Input: dimensioned drawing with shaded views. Units: mm. Origin: part minimum x, y, z. A direction names the side the tool comes from. Round coordinates to 2 decimals unless told otherwise and drop trailing zeros. Loops run counter-clockwise (first coordinate to the right, second up) from the corner with the lowest first, then second, coordinate; pieces in that order, holes last. Notation, with made-up numbers: M -13,64 L 3,64 A15 ccw 3,84 Z; hole C -12,27 d10. An arc over 180 degrees is marked long. Write each question's results on one line, items separated by ' | '. Start each with the question number.
1. Set-up query: the marked faces 1, 2 and 3. Return all of +Z, -Z, +X, -X, +Y, -Y with unobstructed straight access to the full face (end or side cutting, diameter ignored); none if empty.
2. Section C-C on z = 12. Output: boundary loops of the cut face in (x, y).
3. Draft query along Y for the marked faces 4, 5 and 6. Return one class per face: released by +Y, released by -Y, zero draft, split by the parting line, or undercut.
4. Ray query, line 1 (X direction, y = 38, z = 14.5); line 2 (Y direction, x = 10.5, z = 7); line 3 (Y direction, x = 40, z = 13.5) (1 decimal). Return the intervals inside material, ascending.
5. Section A-A on y = 40. Output: boundary loops of the cut face in (x, z).
6. Section D-D on y = 11. Output: boundary loops of the cut face in (x, z), and give its area (3 significant figures).
7. Contact query for flat-ended pins moving along their axis: pin 1 Ø10 at (x, y) = (37.13, 40) entering from -Z; pin 2 Ø3 at (x, z) = (19, 6.5) entering from -Y. Output: stop coordinate, or through.
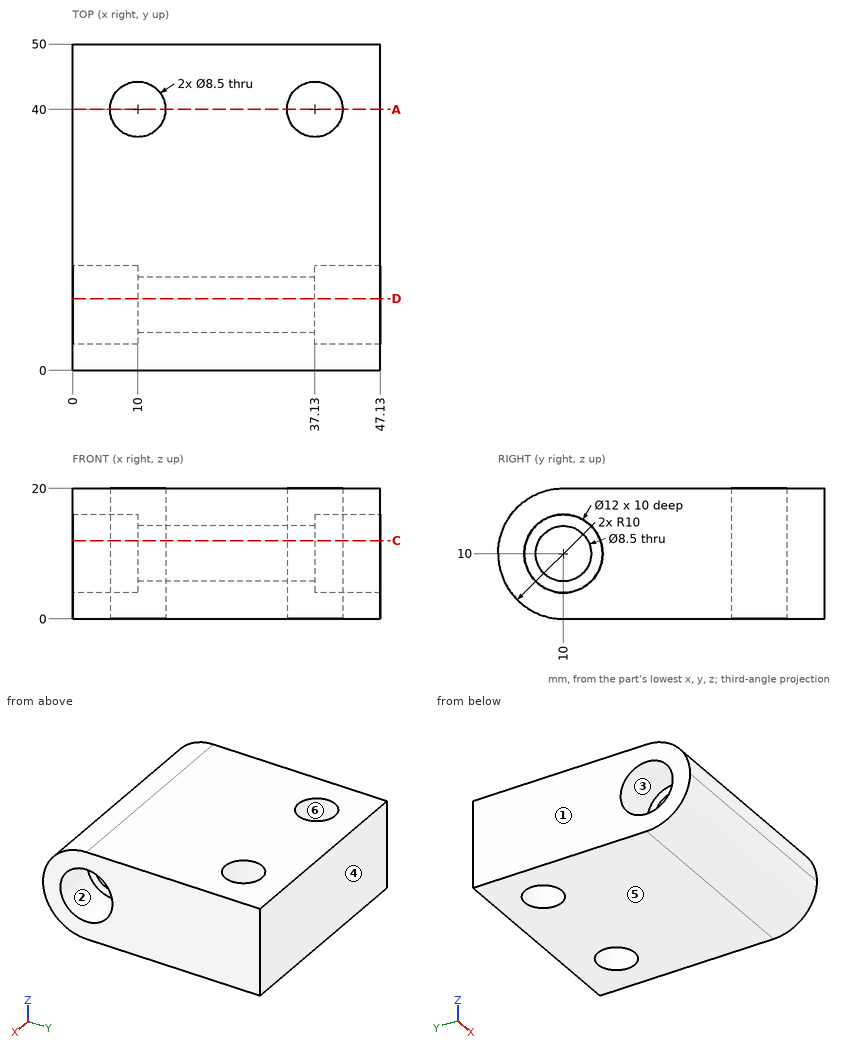
Taken from the geometry:
1) face 1: +Z, -Z, -X, +Y, -Y | face 2: +X | face 3: -X
2) outline: M 0,0.2 L 47.13,0.2 L 47.13,4.34 L 37.13,4.34 L 37.13,6.25 L 10,6.25 L 10,4.34 L 0,4.34 Z; M 0,15.66 L 10,15.66 L 10,13.75 L 37.13,13.75 L 37.13,15.66 L 47.13,15.66 L 47.13,50 L 0,50 Z; hole C 10,40 d8.5; hole C 37.13,40 d8.5
3) face 4: released by +Y | face 5: zero draft | face 6: undercut
4) line 1: 0 to 6.25, 13.75 to 33.38, 40.88 to 47.13 | line 2: 0.46 to 6.99, 13.01 to 35.78, 44.22 to 50 | line 3: 0.6 to 5.1, 14.9 to 36.9, 43.1 to 50
5) outline: M 0,0 L 5.75,0 L 5.75,20 L 0,20 Z; M 14.25,0 L 32.88,0 L 32.88,20 L 14.25,20 Z; M 41.38,0 L 47.13,0 L 47.13,20 L 41.38,20 Z
6) outline: M 0,0 L 47.13,0 L 47.13,4.08 L 37.13,4.08 L 37.13,5.87 L 10,5.87 L 10,4.08 L 0,4.08 Z; M 0,15.92 L 10,15.92 L 10,14.13 L 37.13,14.13 L 37.13,15.92 L 47.13,15.92 L 47.13,20 L 0,20 Z | area: 482 mm^2
7) pin 1: z = 0 | pin 2: y = 0.2
